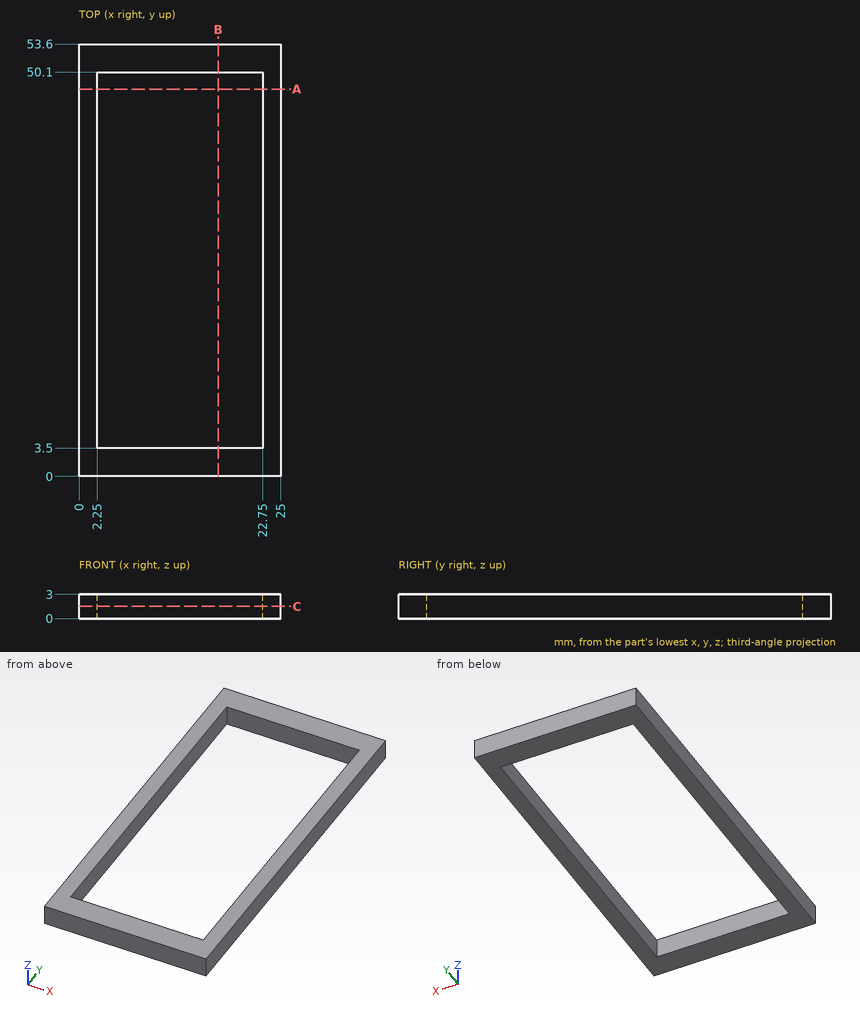
Check sheet for the drawn part. Datum: minimum x, y, z corner. Units: mm. Round coordinates to 2 decimals unless told otherwise and drop trailing zeros. Order: outer loops, then holes, each group sorted by start corner. A loop starts at its lowest first (then second) coordinate and runs counter-clockwise, first axis right, second up. Notation, with made-up numbers: M 50,-21 L 103,-21 A11 ccw 103,-7 Z; hole C 87.5,37.25 d1. An arc over 180 degrees is marked long. Write each question's results on one line, items separated by ' | '. Start each with the question number.
1. Go/stop test with flat-tipped pins: P1, Ø1, axis at y = 16.5, z = 1, coming from the -X side; P2, Ø12, axis at x = 16.5, y = 33, coming from the +Z side. Record where each tip stops, or that it passes through.
2. Cross-section at A-A on y = 48. Record the boundary of the cut face in (x, z), plus the area to 3 significant figures.
3. Cross-section at B-B on x = 17.25. Record the boundary of the cut face in (y, z), plus the area to 3 significant figures.
4. Material ranges on L1, parallel to Y at x = 3, z = 2.3; L2, parallel to X at y = 8.5, z = 2.1, recorded low to high. Write a range as from..to.
5. Cross-section at C-C on z = 1.5. Record the boundary of the cut face in (x, y), plus the area to 3 significant figures.
Resolved:
1) P1: x = 0 | P2: through
2) outline: M 0,0 L 2.25,0 L 2.25,3 L 0,3 Z; M 22.75,0 L 25,0 L 25,3 L 22.75,3 Z | area: 13.5 mm2
3) outline: M 0,0 L 3.5,0 L 3.5,3 L 0,3 Z; M 50.1,0 L 53.6,0 L 53.6,3 L 50.1,3 Z | area: 21.0 mm2
4) L1: 0..3.5, 50.1..53.6 | L2: 0..2.25, 22.75..25
5) outline: M 0,0 L 25,0 L 25,53.6 L 0,53.6 Z; hole M 2.25,3.5 L 22.75,3.5 L 22.75,50.1 L 2.25,50.1 Z | area: 385 mm2
